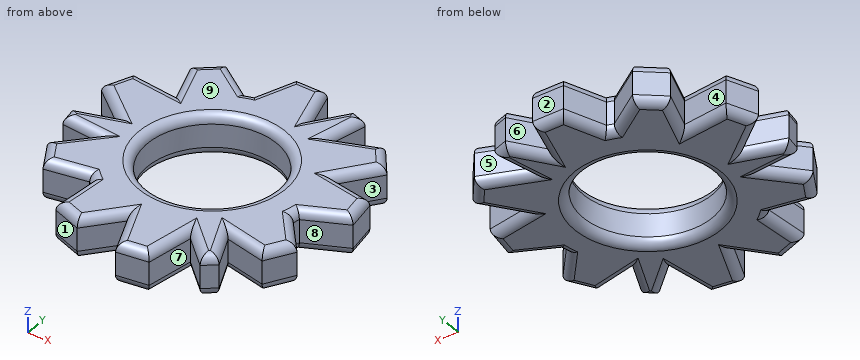
from build123d import *

# Parameters (mm, degrees)
F0_R     = 11.2
F1_DEPTH = 7
F2_R     = 1.5


with BuildPart() as f1:
    # F0 (on Top) → F1 (new body)
    with BuildSketch(Plane.XY):
        with BuildLine():
            Line((-2.554869, 23.895517), (-5.062115, 16.96069))
            ThreePointArc((-5.062115, 16.96069), (-5.619032, 16.784412), (-6.16983, 16.589852))
            Line((-6.16983, 16.589852), (-12.572387, 20.99502))
            Line((-12.572387, 20.99502), (-16.716925, 17.517339))
            Line((-16.716925, 17.517339), (-14.179966, 10.593327))
            Line((-14.179966, 10.593327), (-22.082106, 11.478296))
            Line((-22.082106, 11.478296), (-24.111726, 6.463109))
            Line((-24.111726, 6.463109), (-17.656009, 1.24714))
            Line((-17.656009, 1.24714), (-24.162371, -0.823202))
            Line((-24.162371, -0.823202), (-23.685021, -3.496856))
            Line((-23.685021, -3.496856), (-17.21945, -4.096405))
            Line((-17.21945, -4.096405), (-22.121846, -9.474873))
            Line((-22.121846, -9.474873), (-19.41669, -14.16034))
            Line((-19.41669, -14.16034), (-12.157331, -12.864265))
            ThreePointArc((-12.157331, -12.864265), (-11.726211, -13.258431), (-11.282319, -13.638155))
            Line((-11.282319, -13.638155), (-11.896027, -21.385516))
            Line((-11.896027, -21.385516), (-6.811998, -23.235951))
            Line((-6.811998, -23.235951), (-2.084107, -17.576874))
            Line((-2.084107, -17.576874), (1.100557, -24.862813))
            Line((1.100557, -24.862813), (6.458647, -24.112921))
            Line((6.458647, -24.112921), (7.747949, -15.914122))
            Line((7.747949, -15.914122), (12.7941, -20.513626))
            Line((12.7941, -20.513626), (14.870876, -18.763402))
            Line((14.870876, -18.763402), (12.157316, -12.864279))
            Line((12.157316, -12.864279), (19.266404, -14.420644))
            Line((19.266404, -14.420644), (21.971559, -9.735177))
            Line((21.971559, -9.735177), (17.219446, -4.096425))
            ThreePointArc((17.219446, -4.096425), (17.345243, -3.525981), (17.452148, -2.951697))
            Line((17.452148, -2.951697), (24.468414, 0.390496))
            Line((24.468414, 0.390496), (23.528923, 5.718612))
            Line((23.528923, 5.718612), (16.264073, 6.983547))
            Line((16.264073, 6.983547), (20.981549, 13.384517))
            Line((20.981549, 13.384517), (17.653079, 17.649813))
            Line((17.653079, 17.649813), (9.908059, 14.666982))
            Line((9.908059, 14.666982), (11.368272, 21.336828))
            Line((11.368272, 21.336828), (8.814145, 22.260258))
            Line((8.814145, 22.260258), (5.062135, 16.960684))
            Line((5.062135, 16.960684), (2.855442, 23.895517))
            Line((2.855442, 23.895517), (-2.554869, 23.895517))
        make_face()
        Circle(F0_R, mode=Mode.SUBTRACT)
    extrude(amount=F1_DEPTH)

    # F2
    f2_edges = [f1.edges().sort_by_distance(p)[0] for p in [
        (17.345243, -3.525981, 0),
        (20.960281, -1.2806, 0),
        (23.998669, 3.054554, 0),
        (19.896498, 6.35108, 0),
        (18.622811, 10.184032, 0),
        (19.317314, 15.517165, 0),
        (13.780569, 16.158397, 0),
        (10.638166, 18.001905, 0),
        (10.091208, 21.798543, 0),
        (6.93814, 19.610471, 0),
        (3.958788, 20.4281, 0),
        (0.150286, 23.895517, 0),
        (-3.808492, 20.428103, 0),
        (-5.619032, 16.784412, 0),
        (-9.371108, 18.792436, 0),
        (-14.644656, 19.25618, 0),
        (-15.448445, 14.055333, 0),
        (-18.131036, 11.035811, 0),
        (-23.096916, 8.970702, 0),
        (-20.883867, 3.855124, 0),
        (-20.90919, 0.211969, 0),
        (-23.923696, -2.160029, 0),
        (-20.452236, -3.79663, 0),
        (-19.670648, -6.785639, 0),
        (-20.769268, -11.817607, 0),
        (-15.787011, -13.512302, 0),
        (-11.726211, -13.258431, 0),
        (-11.589173, -17.511836, 0),
        (-9.354013, -22.310734, 0),
        (-4.448053, -20.406413, 0),
        (-0.491775, -21.219843, 0),
        (3.779602, -24.487867, 0),
        (7.103298, -20.013522, 0),
        (10.271024, -18.213874, 0),
        (13.832488, -19.638514, 0),
        (13.514096, -15.813841, 0),
        (15.71186, -13.642461, 0),
        (20.618982, -12.07791, 0),
        (19.595502, -6.915801, 0),
        (-11.2, 0, 0),
        (17.345243, -3.525981, 7),
        (20.960281, -1.2806, 7),
        (23.998669, 3.054554, 7),
        (19.896498, 6.35108, 7),
        (18.622811, 10.184032, 7),
        (19.317314, 15.517165, 7),
        (13.780569, 16.158397, 7),
        (10.638166, 18.001905, 7),
        (10.091208, 21.798543, 7),
        (6.93814, 19.610471, 7),
        (3.958788, 20.4281, 7),
        (0.150286, 23.895517, 7),
        (-3.808492, 20.428103, 7),
        (-5.619032, 16.784412, 7),
        (-9.371108, 18.792436, 7),
        (-14.644656, 19.25618, 7),
        (-15.448445, 14.055333, 7),
        (-18.131036, 11.035811, 7),
        (-23.096916, 8.970702, 7),
        (-20.883867, 3.855124, 7),
        (-20.90919, 0.211969, 7),
        (-23.923696, -2.160029, 7),
        (-20.452236, -3.79663, 7),
        (-19.670648, -6.785639, 7),
        (-20.769268, -11.817607, 7),
        (-15.787011, -13.512302, 7),
        (-11.726211, -13.258431, 7),
        (-11.589173, -17.511836, 7),
        (-9.354013, -22.310734, 7),
        (-4.448053, -20.406413, 7),
        (-0.491775, -21.219843, 7),
        (3.779602, -24.487867, 7),
        (7.103298, -20.013522, 7),
        (10.271024, -18.213874, 7),
        (13.832488, -19.638514, 7),
        (13.514096, -15.813841, 7),
        (15.71186, -13.642461, 7),
        (20.618982, -12.07791, 7),
        (19.595502, -6.915801, 7),
        (-11.2, 0, 7),
    ]]
    fillet(f2_edges, radius=F2_R)


solid = f1.part
Design review of the part built by this model. Coordinates are the model's own, in mm. Face numbers are marked on the shaded views. A direction names the side the tool comes from. Give positions to 0.01 mm unless a question says otherwise; leave off trailing zeros.
1. To check wall thickness, follow L1, parallel to Y at x = 19.5, z = 0.75; L2, parallel to Y at x = 18, z = 1.5; L3, parallel to Y at x = 0, z = 2.75. State the ranges of each line that lie inside material, in increasing order.
Solution:
L1: y = -13.61 to -7.11, -1.75 to 6.22, 11.71 to 14.96
L2: y = -14.14 to -5.02, -2.69 to 6.68, 9.34 to 17.21
L3: y = -22.34 to -11.2, 11.2 to 23.9
2. Mouldability with a two-part tool opening along X and no side actions: class the marked faces 1, 2, 3 and 4 as +X half, -X half, draft (parallel to the pull), parting line (faces both ways), or undercut.
Solution:
face 1: -X half
face 2: draft
face 3: +X half
face 4: undercut
3. For pin 1 Ø2 at (y, z) = (2, 1) entering from -X; pin 2 Ø1.5 at (x, z) = (-15.5, 3) entering from +Y; pin 3 Ø2 at (y, z) = (-16.5, 1.5) entering from +X, all flat-tipped, find the tip position at first contact; note any pin that passes through.
Solution:
pin 1: stops at x = -19.75
pin 2: stops at y = 19.17
pin 3: stops at x = 14.29
4. Tool access review of the marked faces 5, 6, 7, 8 and 9: name each direction out of +Z, -Z, +X, -X, +Y, -Y from which nothing blocks a thin tool from reaching the whole face with its end or side.
Solution:
face 5: +Z, -Z
face 6: +Z, -Z, +Y
face 7: +Z, -Z, -Y
face 8: +Z, -Z, +X
face 9: +Z, +X, -X, +Y, -Y
